Geometry: final body of the model. Coordinates: model frame, mm. A direction names the side the tool comes from. Coordinates: 2 decimals unless noted, no trailing zeros. Order: outer loops, then holes, each group sorted by start corner. A loop starts at its lowest first (then second) coordinate and runs counter-clockwise, first axis right, second up. Notation, with made-up numbers: (83, 76) -> (125, 76) arc R23 ccw to (125, 94) -> close; hole circle Ø10 at (65, 18.5). An arc over 180 degrees is marked (long way). Use one line per item in the form item = value.
Autodesk Inventor part; units mm, degrees
ref_plane "YZ Plane" through (0, 0, 0) normal (1, 0, 0) x (0, 1, 0)
ref_plane "XZ Plane" through (0, 0, 0) normal (0, 1, 0) x (-1, 0, 0)
ref_plane "XY Plane" through (0, 0, 0) normal (0, 0, 1) x (1, 0, 0)
sketch "Sketch1" plane through (0, 0, 0) normal (0, 1, 0) x (-1, 0, 0)
  line L0 (20, 22.5) -> (-20, 22.5)
  line L1 (-20, 22.5) -> (-20, -22.5)
  line L2 (-20, -22.5) -> (20, -22.5)
  line L3 (20, -22.5) -> (20, 22.5)
  point P0 (0, 0)
  point P1 (-20, 0)
  point P2 (20, 0)
  point P3 (0, 22.5)
  point P4 (0, -22.5)
  dimension "d2" = 45
  dimension "d3" = 40
extrude "Extrusion1" add sketch "Sketch1" along normal blind 3
sketch "Sketch2" plane through (0, 3, 0) normal (0, 1, 0) x (1, 0, 0)
  circle A0 centre (0, 0) radius 2.5
  dimension "d4" = 5
extrude "Extrusion2" add sketch "Sketch2" along normal blind 40
fillet "Fillet1" radius 7 1 edges at (-2.5, 3, 0)
sketch "Sketch3" plane through (0, 3, 0) normal (0, 1, 0) x (1, 0, 0)
  circle A0 centre (0, 0) radius 13
  circle A1 centre (0, 0) radius 15
  dimension "d8" = 26
  dimension "d9" = 30
extrude "Extrusion3" add sketch "Sketch3" along normal blind 10
sketch "Sketch4" plane through (0, 3, 0) normal (0, 1, 0) x (1, 0, 0)
  line L0 (20, 22.5) -> (-20, 22.5)
  line L1 (20, -22.5) -> (20, 22.5)
  line L2 (-20, -22.5) -> (20, -22.5)
  line L3 (-20, 22.5) -> (-20, -22.5)
  point P0 (0, 0)
  point P1 (15, -17.5)
  point P2 (15, 17.5)
  point P3 (-15, 17.5)
  point P4 (-15, -17.5)
  dimension "d12" = 5
  dimension "d13" = 5
  dimension "d14" = 5
  dimension "d15" = 5
  dimension "d16" = 5
  dimension "d17" = 5
  dimension "d18" = 5
  dimension "d19" = 5
hole "Hole1" at (15, 3, 17.5) at (15, 3, -17.5) at (-15, 3, -17.5) at (-15, 3, 17.5) direction (0, -1, 0) diameter 2 end through all
fillet "Fillet2" radius 3 1 edges at (-15, 3, 0)
fillet "Fillet3" radius 2 1 edges at (-13, 3, 0)
fillet "Fillet4" radius 4 4 edges at (20, 1.5, 22.5) (20, 1.5, -22.5) (-20, 1.5, 22.5) (-20, 1.5, -22.5)
fillet "Fillet5" radius 2 8 edges at (-18.8284, 3, 21.3284) (0, 3, 22.5) (18.8284, 3, 21.3284) (20, 3, 0) (18.8284, 3, -21.3284) (0, 3, -22.5) (-18.8284, 3, -21.3284) (-20, 3, 0)
fillet "Fillet6" radius 2 1 edges at (-15, 13, 0)
properties part number "Upper_part"
1) Section B-B, the plane y = 23.5. Output: boundary loops of the cut face in (x, z), and give its area (3 significant figures).
Results found:
outline = circle Ø5 at (0, 0)
area = 19.6 mm2
2) Access query for faces 4 (the flat face through (7, 3, 17)), 5 (the cylindrical face through (18.797, 0.507, 21.359)). Directions: +Z, -Z, +X, -X, +Y, -Y. A direction counts if a zero-diameter tool reaches every point of the face in a straight line with its end or side. Return the directions, or none.
Results found:
face_4 = +Y
face_5 = +Z, +X, +Y, -Y
3) Section A-A, the plane y = 4. Output: boundary loops of the cut face in (x, z).
Results found:
outline = circle Ø31.53 at (0, 0); circle Ø11.79 at (0, 0); hole circle Ø25.46 at (0, 0)
4) Pull-direction query (Z, two-part tool) for faces 1 (the cylindrical face through (-10.316, 8.944, -7.91)), 2 (the cylindrical face through (-14.985, 8.465, 0.66)), 3 (the cylindrical face through (-19.4, 2.43, 0.26)); classes: released by +Z, released by -Z, zero draft, split by the parting line, or undercut.
Results found:
face_1 = undercut
face_2 = split by the parting line
face_3 = zero draft
5) Material intervals for probe 1 along Z at (x, y) = (-15, 1); probe 2 along X at (y, z) = (10.75, 0); probe 3 along X at (y, z) = (2.05, 17.5), sorted ascending. Write a range as from..to.
Results found:
probe_1 = -22.5..-18.5, -16.5..16.5, 18.5..22.5
probe_2 = -15..-13, -2.5..2.5, 13..15
probe_3 = -19.7..-16, -14..14, 16..19.7
6) Section C-C, the plane y = 8.5. Output: boundary loops of the cut face in (x, z).
Results found:
outline = circle Ø30 at (0, 0); circle Ø5.33 at (0, 0); hole circle Ø26 at (0, 0)
7) Contact query for flat-ended pins moving along their axis: P1, Ø2, axis at x = 10, z = -10.5, coming from the +Y side; P2, Ø1.6, axis at x = -15, z = 17.5, coming from the -Y side; P3, Ø4, axis at x = 3.5, z = 6, coming from the +Y side; P4, Ø1.5, axis at x = 9.5, y = 10, coming from the +Z side. Output: stop coordinate, or through.
Results found:
P1 = 12.94
P2 = through
P3 = 4.68
P4 = 12.18
